```python
from build123d import *


with BuildPart() as f2:
    # F2: sweep along a path in F1
    with BuildLine(Plane.XY) as f2_path:
        Line((0, 0), (0, 2000))
    # F0 (on Front) → F2 (sweep)
    with BuildSketch(Plane.XZ):
        Polygon((125, 0), (139.142136, 0), (29.142136, 110), (-29.142136, 110), (-139.142136, 0), (-125, 0), (-25, 100), (25, 100), align=None)
    sweep(path=f2_path.line)


solid = f2.part
```
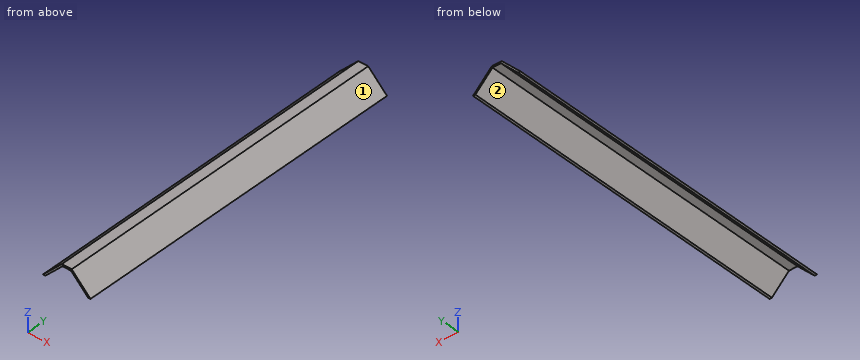
Work out the finished part from the listing and answer in its coordinate system (mm). Face numbers are marked on the shaded views. Coordinates: 2 decimals unless noted, no trailing zeros. Write each loop counter-clockwise with the first axis right and the second up, starting at its lowest first coordinate (ties: lowest second). Pieces come first, ordered by that corner, then holes. Notation, with made-up numbers: (86, 1.25) - (129, 1.25) arc R5 cw to (129, 10.25) - close; hole circle Ø4 at (-34.5, 72.25). An arc over 180 degrees is marked (long way). Answer as a JSON object with one key per item and string values.
Q1. Consider L1, parallel to Z at x = -8.5, y = 654; L2, parallel to X at y = 870.5, z = 85.5; L3, parallel to X at y = 1234, z = 65.5. Determine where each line is inside the solid, lowest interval first. Write a range as from..to.
Results list:
{"L1": "z = 100..110", "L2": "x = -53.64..-39.5, 39.5..53.64", "L3": "x = -73.64..-59.5, 59.5..73.64"}
Q2. Find section C-C (x = -7.5). Write down the section's boundary in (y, z).
Results list:
{"outline": "(0, 100) - (2000, 100) - (2000, 110) - (0, 110) - close"}
Q3. Find section A-A (y = 1822). Write down the section's boundary in (x, z).
Results list:
{"outline": "(-139.14, 0) - (-125, 0) - (-25, 100) - (25, 100) - (125, 0) - (139.14, 0) - (29.14, 110) - (-29.14, 110) - close"}
Q4. For a pull along X with two mould halves and no side action, classify the marked faces 1 and 2 as pulls with the +X half, pulls with the -X half, needs draft (parallel to the pull), parting line crosses it, or undercut.
Results list:
{"face 1": "pulls with the +X half", "face 2": "undercut"}
Q5. Find section B-B (z = 41). Write down the section's boundary in (x, y), plus the area to 3 significant figures.
Results list:
{"outline": "(-98.14, 0) - (-84, 0) - (-84, 2000) - (-98.14, 2000) - close; (84, 0) - (98.14, 0) - (98.14, 2000) - (84, 2000) - close", "area": "56,600 mm^2"}
Q6. Given pin 1 Ø6 at (y, z) = (433.5, 20.5) entering from +X; pin 2 Ø2 at (x, y) = (-34.5, 348.5) entering from +Z; pin 3 Ø8 at (y, z) = (1290, 73.5) entering from +X, each flat-ended and moving along its own axis, determine where each tip first touches the part or whether it passes through.
Results list:
{"pin 1": "stops at x = 121.64", "pin 2": "stops at z = 105.64", "pin 3": "stops at x = 69.64"}
